Model file for the job. Use its own axes, mm. A direction names the side the tool comes from. Round coordinates to 2 decimals unless told otherwise and drop trailing zeros. Order: outer loops, then holes, each group sorted by start corner. A loop starts at its lowest first (then second) coordinate and runs counter-clockwise, first axis right, second up. Notation, with made-up numbers: (-30, 9.25) -> (24, 9.25) arc R13 ccw to (24, 19.25) -> close; hole circle Ø4 at (11, 1). An arc over 180 degrees is marked (long way). Answer as CSV lines item,"result".
```python
from build123d import *

# Parameters (mm, degrees)
F0_W     = 1.2707259422
F0_H     = 3
F2_R     = 2.5
F2_R_2   = 2.0207259422
F3_DEPTH = 3


with BuildPart() as f1:
    # F0 (on Front) → F1 (revolve)
    with BuildSketch(Plane.XZ):
        Polygon((-21.4229148179, -4.8091755062), (-21.4229148179, -4.8227669001), (-20.1521888758, -4.8227669001), (-19.6729148179, -4.8227669001), (-19.6729148179, -3.3227669001), (-19.1892255098, -3.125249641), (-19.1892255098, 10.9797158409), (-19.6729148179, 11.1772330999), (-20.1729148179, 11.1772330999), (-20.1729148179, -2.6441119968), align=None)
        with Locations((-20.7875518468, -6.3227669001)):
            Rectangle(F0_W, F0_H)
        Polygon((-21.4229148179, -7.8227669001), (-21.4229148179, -9.8091755062), (-20.9229148179, -9.8091755062), (-19.2720282078, -7.8227669001), (-20.1521888758, -7.8227669001), align=None)
    revolve(axis=Axis((-22.1729148179, 0, 14.5059827045), (0, 0, 1)))

    # F2 (on face) → F3 (join, through all)
    with BuildSketch(Plane(origin=(0, 0, -4.8227669001), x_dir=(1, 0, 0), z_dir=(0, 0, -1))):
        Polygon((-20.1521888758, 3.5), (-24.1936407601, 3.5), (-26.2143667023, 0), (-24.1936407601, -3.5), (-20.1521888758, -3.5), (-18.1314629336, 0), align=None)
        with Locations((-22.1729148179, 0)):
            Circle(F2_R, mode=Mode.SUBTRACT)
        with Locations((-22.1729148179, 0)):
            Circle(F2_R)
        with Locations((-22.1729148179, 0)):
            Circle(F2_R_2, mode=Mode.SUBTRACT)
    extrude(amount=F3_DEPTH)


with BuildPart() as f1_1:
    # F4: moved
    add(f1.part.moved(Location((22.1729148179, 0, 9.8091755062))))


solid = f1_1.part
```
Q1. Mould opens along Z. For faces 4 (the flat face through (3, 1.8, 3.5)), 5 (the flat face through (3, 0, 4.986)), 6 (the flat face through (-1, 2, 20.986)), 7 (the flat face through (3, -1, 1.986)) say: +Z half, -Z half, draft (parallel to the pull), parting line (faces both ways), or undercut.
Checks:
face 4,"draft"
face 5,"undercut"
face 6,"+Z half"
face 7,"-Z half"
Q2. Flat gauge pins, fed straight in: pin 1 (1 mm diameter, centred on x = 0.5, y = 0.5, fed in from +Z); pin 2 (1.5 mm diameter, centred on x = 0.5, z = 15, fed in from +Y); pin 3 (1 mm diameter, centred on y = -2.5, z = 19, fed in from -X). Where does each tip first touch, or does it go through?
Checks:
pin 1,"z = 5.79"
pin 2,"y = 2.98"
pin 3,"x = -2.21"
Q3. Saw through at B-B (z = 3.25). Write the cut outline in (x, y), plus the area to 3 significant figures.
Checks:
outline,"(-4.04, 0) -> (-2.02, -3.5) -> (2.02, -3.5) -> (4.04, 0) -> (2.02, 3.5) -> (-2.02, 3.5) -> close; hole circle Ø1.5 at (0, 0)"
area,"40.7 mm²"
Q4. Saw through at A-A (x = 0). Write the cut outline in (y, z).
Checks:
outline,"(-3.5, 1.99) -> (-2.9, 1.99) -> (-1.25, 0) -> (-0.75, 0) -> (-0.75, 5) -> (-2, 7.17) -> (-2, 20.99) -> (-2.5, 20.99) -> (-2.98, 20.79) -> (-2.98, 6.68) -> (-2.5, 6.49) -> (-2.5, 4.99) -> (-3.5, 4.99) -> close; (0.75, 0) -> (1.25, 0) -> (2.9, 1.99) -> (3.5, 1.99) -> (3.5, 4.99) -> (2.5, 4.99) -> (2.5, 6.49) -> (2.98, 6.68) -> (2.98, 20.79) -> (2.5, 20.99) -> (2, 20.99) -> (2, 7.17) -> (0.75, 5) -> close"
Q5. Saw through at C-C (z = 11.75). Write the cut outline in (x, y).
Checks:
outline,"circle Ø5.97 at (0, 0); hole circle Ø4 at (0, 0)"
Q6. Wall check: L1, parallel to Y at x = 0, z = 3.2; L2, parallel to Y at x = 0, z = 14.75; L3, parallel to X at y = 1, z = 13.5. Give the ranges that are in metal, low to high. Write a range as [from, to].
Checks:
L1,"[-3.5, -0.75], [0.75, 3.5]"
L2,"[-2.98, -2], [2, 2.98]"
L3,"[-2.81, -1.73], [1.73, 2.81]"
Q7. Tool access for faces 1 (the flat face through (-3, -1.8, 3.5)), 2 (the cylindrical face through (2.756, -1.143, 13.835)), 3 (the cylindrical face through (-0.54, -2.44, 5.75)): list every direction of +Z, -Z, +X, -X, +Y, -Y with a clear straight run to the whole face (end or side of a thin tool).
Checks:
face 1,"+Z, -Z, -X, -Y"
face 2,"+Z"
face 3,"none"
